Work out the finished part from the listing and answer in its coordinate system (mm). A direction names the side the tool comes from. Give positions to 0.01 mm unless a question says otherwise; leave off trailing zeros. Order: outer loops, then holes, each group sorted by start corner. A loop starts at its lowest first (then second) coordinate and runs counter-clockwise, first axis right, second up. Notation, with made-up numbers: (44, -22) - (50, -22) arc R34 ccw to (50, 8) - close; hole circle Ø5 at (27, 62). An arc over 180 degrees is marked (long way). Write each question's results on one line, items separated by ' | '.
from build123d import *

# Parameters (mm, degrees)
SZKIC2_R                        = 1.75
WYTNIJ_WYCI_GNI_CIE1_DEPTH      = 12
WYTNIJ_WYCI_GNI_CIE1_DEPTH_BACK = 12
SFAZOWANIE1_SIZE                = 1


with BuildPart() as part:
    # Szkic1 → Obrót1 (revolve)
    with BuildSketch(Plane.XY):
        Polygon((0, 0), (0, 11), (4, 11), (4, 8), (52, 8), (52, 0), align=None)
    revolve(axis=Axis((52, 0, 0), (-1, 0, 0)))

    # Szkic2 → Wytnij-wyciągnięcie1 (cut, two sides)
    with BuildSketch(Plane(origin=(0, 0, 0), x_dir=(1, 0, 0), z_dir=(0, 1, 0))) as wytnij_wyci_gni_cie1_sk:
        with Locations((45.75, 0)):
            Circle(SZKIC2_R)
    extrude(amount=WYTNIJ_WYCI_GNI_CIE1_DEPTH, mode=Mode.SUBTRACT)
    extrude(wytnij_wyci_gni_cie1_sk.sketch, amount=-WYTNIJ_WYCI_GNI_CIE1_DEPTH_BACK, mode=Mode.SUBTRACT)

    # Sfazowanie1
    sfazowanie1_edges = [part.edges().sort_by_distance(p)[0] for p in [
        (52, -8, 0),
        (0, -11, 0),
    ]]
    chamfer(sfazowanie1_edges, length=SFAZOWANIE1_SIZE)


solid = part.part
1. Determine the mould class of faces 1 (the face through (4, -2, 8)), 2 (the face through (0, 0, 0)), 3 (the face through (2.52, -2.38, 10.74)) for opening direction X: +X half, -X half, draft (parallel to the pull), parting line (faces both ways), or undercut.
Answer list:
face 1: +X half | face 2: -X half | face 3: draft
2. A cutting plane is placed at A-A, the plane z = 0. Write down the section's boundary in (x, y).
Answer list:
outline: (0, -10) - (1, -11) - (4, -11) - (4, -8) - (44, -8) - (44, 8) - (4, 8) - (4, 11) - (1, 11) - (0, 10) - close; (47.5, -8) - (51, -8) - (52, -7) - (52, 7) - (51, 8) - (47.5, 8) - close
3. A cutting plane is placed at C-C, the plane x = 45.75. Write down the section's boundary in (y, z), then the cut area to 3 significant figures.
Answer list:
outline: (-7.81, -1.75) arc R8 ccw to (7.81, -1.75) - close; (-7.81, 1.75) - (7.81, 1.75) arc R8 ccw to start | area: 146 mm^2
4. A cutting plane is placed at B-B, the plane x = 7.5. Write down the section's boundary in (y, z), then the cut area to 3 significant figures.
Answer list:
outline: circle Ø16 at (0, 0) | area: 201 mm^2
5. A tool of negligible diameter and unlimited length cuts with its end or side. For faces 4 (the face through (52, 0, 0)), 5 (the face through (27.83, -1.73, 7.81)), from which of +Z, -Z, +X, -X, +Y, -Y can it reach the whole face along a straight path? Write none if from no direction.
Answer list:
face 4: +Z, -Z, +X, +Y, -Y | face 5: +X
6. Given P1, Ø4, axis at x = 45.75, z = 0, coming from the -Y side; P2, Ø12, axis at x = 27.5, z = -8, coming from the -Y side; P3, Ø5, axis at x = 14, z = 1.5, coming from the +Y side; P4, Ø3, axis at x = 45.75, z = 0, coming from the -Y side, each flat-ended and moving along its own axis, determine where each tip first touches the part or whether it passes through.
Answer list:
P1: y = -8 | P2: y = -7.75 | P3: y = 8 | P4: through
7. Straight lines are drawn through the part: line 1 (X direction, y = -4, z = 0); line 2 (Z direction, x = 45.75, y = -2.75); line 3 (X direction, y = 1, z = -9.25). For each, find the intervals that lie inside material, in ascending order. Write a range as [from, to].
Answer list:
line 1: [0, 44], [47.5, 52] | line 2: [-7.51, -1.75], [1.75, 7.51] | line 3: [0, 4]
